Verification items for the finished model (mm, model axes). Face numbers are marked on the shaded views. A direction names the side the tool comes from. Round coordinates to 2 decimals unless told otherwise and drop trailing zeros. Order: outer loops, then holes, each group sorted by start corner. A loop starts at its lowest first (then second) coordinate and runs counter-clockwise, first axis right, second up. Notation, with made-up numbers: (-5, -17.75) -> (27, -17.75) arc R19 cw to (27, -11.75) -> close; hole circle Ø7 at (73, -21). An arc over 180 degrees is marked (long way). Return JSON: item names as keys, results as strings. Group by question number.
1) Draft check along X on the marked faces 3 and 4. Enter one of: pulls with the +X half, pulls with the -X half, needs draft (parallel to the pull), parting line crosses it, or undercut.
2) Depth check by flat-ended pin: pin 1 (5 mm diameter, centred on x = -29.44, z = 33.26, fed in from -Y). Enter the tip coordinate at first touch or a pass-through.
3) Section check C-C on y = 5.25. State how many separate pieces and enclosed holes the cut face has, plus the area to 3 significant figures.
4) Tool access check on the marked faces 1 and 2. Record the directions out of +Z, -Z, +X, -X, +Y, -Y that give a thin tool (end or side, any length) a straight path to the whole face; none if there is none.
5) Section check D-D on x = -29.17. Enter the section's corners in (y, z), plus the area to 3 significant figures.
6) Section check A-A on z = 8.13. Enter the section's corners in (x, y).
7) Scan lines: L1, parallel to Z at x = -29.17, y = 3.25; L2, parallel to X at y = 3.25, z = 33.5; L3, parallel to Z at x = -37.3, y = 5.25. Record each from-to range of solid material in increasing order.
8) Section check B-B on z = 0. Enter the section's corners in (x, y).
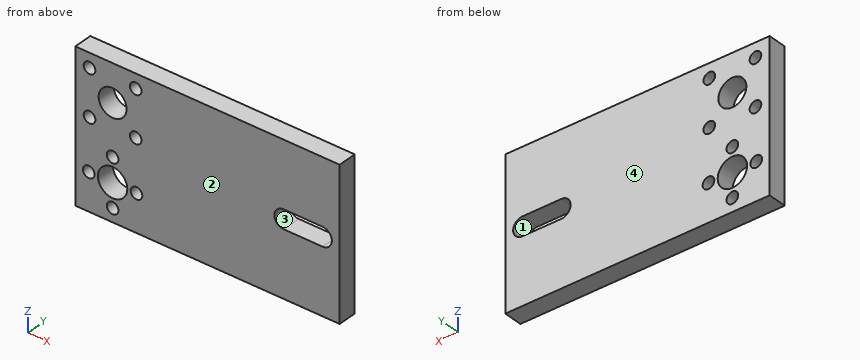
```python
from build123d import *

# Parameters (mm, degrees)
SKETCH1_W           = 90
SKETCH1_H           = 50.8
SKETCH1_R           = 5
SKETCH1_R_2         = 1.984375
SKETCH1_R_3         = 4.7625
BOSS_EXTRUDE1_DEPTH = 6.35


with BuildPart() as part:
    # Sketch1 → Boss-Extrude1 (new body)
    with BuildSketch(Plane(origin=(0, 0, 0), x_dir=(1, 0, 0), z_dir=(0, 1, 0))):
        with Locations((-5, -12.7)):
            Rectangle(SKETCH1_W, SKETCH1_H)
        with Locations((-37.3, 0)):
            Circle(SKETCH1_R, mode=Mode.SUBTRACT)
        with Locations((-37.3, -8.13)):
            Circle(SKETCH1_R_2, mode=Mode.SUBTRACT)
        with Locations((-45.43, 0)):
            Circle(SKETCH1_R_2, mode=Mode.SUBTRACT)
        with Locations((-37.3, 8.13)):
            Circle(SKETCH1_R_2, mode=Mode.SUBTRACT)
        with Locations((-29.17, 0)):
            Circle(SKETCH1_R_2, mode=Mode.SUBTRACT)
        with Locations((-37.3, -25.4)):
            Circle(SKETCH1_R_3, mode=Mode.SUBTRACT)
        with Locations((-45.157724106, -17.542275894)):
            Circle(SKETCH1_R_2, mode=Mode.SUBTRACT)
        with Locations((-29.442275894, -17.542275894)):
            Circle(SKETCH1_R_2, mode=Mode.SUBTRACT)
        with Locations((-29.442275894, -33.257724106)):
            Circle(SKETCH1_R_2, mode=Mode.SUBTRACT)
        with Locations((-45.157724106, -33.257724106)):
            Circle(SKETCH1_R_2, mode=Mode.SUBTRACT)
        with BuildLine():
            Line((20.945, -9.525), (34.155, -9.525))
            ThreePointArc((34.155, -9.525), (37.33, -12.7), (34.155, -15.875))
            Line((34.155, -15.875), (20.945, -15.875))
            ThreePointArc((20.945, -15.875), (17.77, -12.7), (20.945, -9.525))
        make_face(mode=Mode.SUBTRACT)
    extrude(amount=BOSS_EXTRUDE1_DEPTH)


solid = part.part
```
Check result:
{
 "1": {"face 3": "undercut", "face 4": "needs draft"},
 "2": {"pin 1": "y = 0"},
 "3": {"separate pieces": "1", "enclosed holes": "11", "area": "4,210 mm^2"},
 "4": {"face 1": "+Y, -Y", "face 2": "+Z, -Z, +X, -X, -Y"},
 "5": {"outline": "(0, -12.7) -> (6.35, -12.7) -> (6.35, -1.98) -> (0, -1.98) -> close; (0, 1.98) -> (6.35, 1.98) -> (6.35, 15.58) -> (0, 15.58) -> close; (0, 19.51) -> (6.35, 19.51) -> (6.35, 31.29) -> (0, 31.29) -> close; (0, 35.22) -> (6.35, 35.22) -> (6.35, 38.1) -> (0, 38.1) -> close", "area": "247 mm^2"},
 "6": {"outline": "(-50, 0) -> (-39.28, 0) -> (-39.28, 6.35) -> (-50, 6.35) -> close; (-35.32, 0) -> (40, 0) -> (40, 6.35) -> (-35.32, 6.35) -> close"},
 "7": {"L1": "-12.7 to -1.98, 1.98 to 15.58, 19.51 to 31.29, 35.22 to 38.1", "L2": "-50 to -47.13, -43.19 to -31.41, -27.47 to 40", "L3": "-12.7 to -10.11, -6.15 to -5, 5 to 6.15, 10.11 to 20.64, 30.16 to 38.1"},
 "8": {"outline": "(-50, 0) -> (-47.41, 0) -> (-47.41, 6.35) -> (-50, 6.35) -> close; (-43.45, 0) -> (-42.3, 0) -> (-42.3, 6.35) -> (-43.45, 6.35) -> close; (-32.3, 0) -> (-31.15, 0) -> (-31.15, 6.35) -> (-32.3, 6.35) -> close; (-27.19, 0) -> (40, 0) -> (40, 6.35) -> (-27.19, 6.35) -> close"}
}
